Model file for the job. Use its own axes, mm. Face numbers are marked on the shaded views. Give positions to 0.01 mm unless a question says otherwise; leave off trailing zeros. Use CSV: the item, a comma, the result in double quotes. Start each with the question number.
(1) Drill centre lines: probe 1 along Y at (x, z) = (0, 2.1); probe 2 along Z at (x, y) = (145, -32); probe 3 along Y at (x, z) = (-90, 1.6). Where is each one in solid material? Low to high.
(2) Pull direction X, two halves, no side cores. Call the marked faces 1 and 2: pulls with the +X half, pulls with the -X half, needs draft (parallel to the pull), parting line crosses it, or undercut.
(3) Flat gauge pins, fed straight in: pin 1 (3.5 mm diameter, centred on x = 0, y = 30, fed in from +Z); pin 2 (4 mm diameter, centred on x = 27, y = -22, fed in from -Z); pin 3 (0.8 mm diameter, centred on x = -139, z = 1.5, fed in from +Y); pin 4 (4.5 mm diameter, centred on x = 144.5, z = 7, fed in from +Y). Where does each tip first touch, or does it go through?
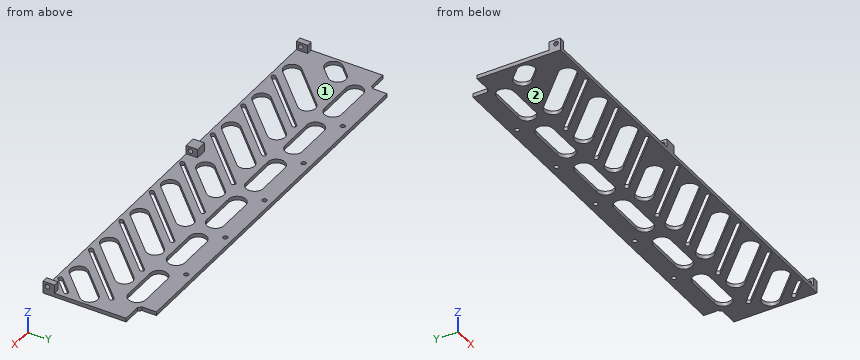
from build123d import *

# Parameters (mm, degrees)
SKETCH_1_W               = 295
SKETCH_1_H               = 70
EXTRUDE_1_DEPTH          = 2.7
CUT_EXTRUDE_5_DEPTH      = 10
CUT_EXTRUDE_1_DEPTH      = 152.619721672
PATTERN_LINEAR_1_COUNT   = 7
PATTERN_LINEAR_1_PITCH   = 35
CUT_EXTRUDE_4_DEPTH      = 152.619721672
SKETCH_5_W               = 4
SKETCH_5_H               = 8
SKETCH_5_W_2             = 8
EXTRUDE_3_DEPTH          = 6
CUT_EXTRUDE_3_DEPTH      = 294.22634602
CUT_EXTRUDE_3_DEPTH_BACK = 294.22634602
SKETCH_7_R               = 1.6
CUT_EXTRUDE_6_DEPTH      = 152.714369787
PATTERN_LINEAR_2_COUNT   = 7
PATTERN_LINEAR_2_PITCH   = 35
PATTERN_LINEAR_3_COUNT   = 3
PATTERN_LINEAR_3_PITCH   = 35
CUT_EXTRUDE_7_DEPTH      = 152.714369787
PATTERN_LINEAR_4_COUNT   = 4
PATTERN_LINEAR_4_PITCH   = 45
PATTERN_LINEAR_5_COUNT   = 3
PATTERN_LINEAR_5_PITCH   = 45
EXTRUDE_4_DEPTH          = 2.7
SKETCH_15_R              = 1.6
CUT_EXTRUDE_8_DEPTH      = 10


with BuildPart() as part:
    # 草图1 → 凸台-拉伸1 (new body)
    with BuildSketch(Plane.XY):
        Rectangle(SKETCH_1_W, SKETCH_1_H)
    extrude(amount=EXTRUDE_1_DEPTH)

    # 草图11 → 切除-拉伸5 (cut)
    with BuildSketch(Plane.XY.offset(2.7)):
        Polygon((-147.5, 35), (-147.5, 23), (-134.5, 23), (-132.5, 25), (-132.5, 35), align=None)
        Polygon((132.5, 35), (147.5, 35), (147.5, 23), (134.5, 23), (132.5, 25), align=None)
    extrude(amount=-CUT_EXTRUDE_5_DEPTH, mode=Mode.SUBTRACT)

    # 草图2 → 切除-拉伸1 (cut, through all)
    with BuildSketch(Plane.XY.offset(2.7)):
        with BuildLine():
            Line((-113.560660172, -30.939339828), (-76.560660172, 6.060660172))
            ThreePointArc((-76.560660172, 6.060660172), (-74.439339828, 6.060660172), (-74.439339828, 3.939339828))
            Line((-74.439339828, 3.939339828), (-111.439339828, -33.060660172))
            ThreePointArc((-111.439339828, -33.060660172), (-113.560660172, -33.060660172), (-113.560660172, -30.939339828))
        make_face()
    cut_extrude_1 = extrude(amount=-CUT_EXTRUDE_1_DEPTH, mode=Mode.SUBTRACT)

    # 阵列(线性)1: 切除-拉伸1 ×7
    with Locations(*[(i * PATTERN_LINEAR_1_PITCH, 0, 0) for i in range(1, PATTERN_LINEAR_1_COUNT)]):
        add(cut_extrude_1, mode=Mode.SUBTRACT)

    # 草图10 → 切除-拉伸4 (cut, through all)
    with BuildSketch(Plane.XY.offset(2.7)):
        with BuildLine():
            Line((131.439339828, -30.939339828), (141.939339828, -20.439339828))
            ThreePointArc((141.939339828, -20.439339828), (144.060660172, -20.439339828), (144.060660172, -22.560660172))
            Line((144.060660172, -22.560660172), (133.560660172, -33.060660172))
            ThreePointArc((133.560660172, -33.060660172), (131.439339828, -33.060660172), (131.439339828, -30.939339828))
        make_face()
    extrude(amount=-CUT_EXTRUDE_4_DEPTH, mode=Mode.SUBTRACT)

    # 草图5 → 凸台-拉伸3 (add)
    with BuildSketch(Plane.XY.offset(2.7)):
        with Locations((-145.5, -31)):
            Rectangle(SKETCH_5_W, SKETCH_5_H)
        with Locations((145.5, -31)):
            Rectangle(SKETCH_5_W, SKETCH_5_H)
        with Locations((-21, -31)):
            Rectangle(SKETCH_5_W_2, SKETCH_5_H)
    extrude(amount=EXTRUDE_3_DEPTH)

    # 草图7 → 切除-拉伸3 (cut, two sides: drawn at the far end of the back side and taken through both)
    with BuildSketch(Plane(origin=(-143.5, 0, 0), x_dir=(0, 0, -1), z_dir=(1, 0, 0)).offset(-CUT_EXTRUDE_3_DEPTH_BACK)):
        with Locations((-5.7, -32)):
            Circle(SKETCH_7_R)
    extrude(amount=CUT_EXTRUDE_3_DEPTH + CUT_EXTRUDE_3_DEPTH_BACK, mode=Mode.SUBTRACT)

    # 草图12 → 切除-拉伸6 (cut, through all)
    with BuildSketch(Plane.XY.offset(2.7)):
        with BuildLine():
            Line((-93.279437252, -21.971825407), (-66.528174593, 4.779437252))
            ThreePointArc((-66.528174593, 4.779437252), (-58.220562748, 4.779437252), (-58.220562748, -3.528174593))
            Line((-58.220562748, -3.528174593), (-84.971825407, -30.279437252))
            ThreePointArc((-84.971825407, -30.279437252), (-93.279437252, -30.279437252), (-93.279437252, -21.971825407))
        make_face()
    cut_extrude_6 = extrude(amount=-CUT_EXTRUDE_6_DEPTH, mode=Mode.SUBTRACT)

    # 阵列(线性)2: 切除-拉伸6 ×7
    with Locations(*[(i * PATTERN_LINEAR_2_PITCH, 0, 0) for i in range(1, PATTERN_LINEAR_2_COUNT)]):
        add(cut_extrude_6, mode=Mode.SUBTRACT)

    # 阵列(线性)3: 切除-拉伸6 ×3
    with Locations(*[(-i * PATTERN_LINEAR_3_PITCH, 0, 0) for i in range(1, PATTERN_LINEAR_3_COUNT)]):
        add(cut_extrude_6, mode=Mode.SUBTRACT)

    # 草图13 → 切除-拉伸7 (cut, through all)
    with BuildSketch(Plane.XY.offset(2.7)):
        with BuildLine():
            Line((-35, 23), (-10, 23))
            ThreePointArc((-10, 23), (-4, 17), (-10, 11))
            Line((-10, 11), (-35, 11))
            ThreePointArc((-35, 11), (-41, 17), (-35, 23))
        make_face()
    cut_extrude_7 = extrude(amount=-CUT_EXTRUDE_7_DEPTH, mode=Mode.SUBTRACT)

    # 阵列(线性)4: 切除-拉伸7 ×4
    with Locations(*[(i * PATTERN_LINEAR_4_PITCH, 0, 0) for i in range(1, PATTERN_LINEAR_4_COUNT)]):
        add(cut_extrude_7, mode=Mode.SUBTRACT)

    # 阵列(线性)5: 切除-拉伸7 ×3
    with Locations(*[(-i * PATTERN_LINEAR_5_PITCH, 0, 0) for i in range(1, PATTERN_LINEAR_5_COUNT)]):
        add(cut_extrude_7, mode=Mode.SUBTRACT)

    # 草图14 → 凸台-拉伸4 (add)
    with BuildSketch(Plane.XY.offset(2.7)):
        with BuildLine():
            Line((-143.779437252, -2.471825407), (-147.5, -6.192388155))
            Line((-147.5, -6.192388155), (-147.5, -22.807611845))
            Line((-147.5, -22.807611845), (-135.471825407, -10.779437252))
            ThreePointArc((-135.471825407, -10.779437252), (-143.779437252, -10.779437252), (-143.779437252, -2.471825407))
        make_face()
        with BuildLine():
            Line((143.471825407, 4.779437252), (135.471825407, -3.220562748))
            ThreePointArc((135.471825407, -3.220562748), (143.779437252, -3.220562748), (143.779437252, -11.528174593))
            Line((143.779437252, -11.528174593), (147.5, -7.807611845))
            Line((147.5, -7.807611845), (147.5, 6.498656448))
            ThreePointArc((147.5, 6.498656448), (145.31969888, 6.028490093), (143.471825407, 4.779437252))
        make_face()
        with BuildLine():
            Line((-14.794155877, -13.486544033), (-23.279437252, -21.971825407))
            ThreePointArc((-23.279437252, -21.971825407), (-23.279437252, -30.279437252), (-14.971825407, -30.279437252))
            Line((-14.971825407, -30.279437252), (-6.486544033, -21.794155877))
            ThreePointArc((-6.486544033, -21.794155877), (-14.794155877, -21.794155877), (-14.794155877, -13.486544033))
        make_face()
    extrude(amount=-EXTRUDE_4_DEPTH)

    # 草图15 → 切除-拉伸8 (cut)
    with BuildSketch(Plane.XY.offset(2.7)):
        with Locations((-90, 30)):
            Circle(SKETCH_15_R)
        with Locations((-45, 30)):
            Circle(SKETCH_15_R)
        with Locations((45, 30)):
            Circle(SKETCH_15_R)
        with Locations((90, 30)):
            Circle(SKETCH_15_R)
        with Locations((0, 30)):
            Circle(SKETCH_15_R)
    extrude(amount=-CUT_EXTRUDE_8_DEPTH, mode=Mode.SUBTRACT)


solid = part.part
Check result:
1,probe 1,"-35 to -26.62, -22.38 to -15.31, 1.31 to 28.4, 31.6 to 35"
1,probe 2,"0 to 4.1, 7.3 to 8.7"
1,probe 3,"-35 to -31.93, -18.69 to -11.62, -7.38 to 28.4, 31.6 to 35"
2,face 1,"undercut"
2,face 2,"needs draft"
3,pin 1,"z = 2.7"
3,pin 2,"z = 0"
3,pin 3,"y = 23"
3,pin 4,"y = -27"
